from build123d import *

# Parameters (mm, degrees)
F0_R          = 9.525
F1_DEPTH      = 127
F2_R          = 9.525
F3_DEPTH      = 38.1
F3_DEPTH_BACK = 38.1


with BuildPart() as f1:
    # F0 (on Front) → F1 (new body)
    with BuildSketch(Plane.XZ):
        Polygon((-9.525, -23.880164), (-9.525, -36.580164), (9.525, -36.580164), (9.525, -23.880164), (19.05, -23.880164), (19.05, 0), (19.05, 25.4), (0, 25.4), (-19.05, 25.4), (-19.05, 0), (-19.05, -23.880164), align=None)
        Circle(F0_R, mode=Mode.SUBTRACT)
    extrude(amount=F1_DEPTH)

    # F2 (on Right) → F3 (cut, two sides)
    with BuildSketch(Plane.YZ) as f3_sk:
        with Locations((-32.103937, 0)):
            Circle(F2_R)
        with Locations((-95.37492, 0)):
            Circle(F2_R)
    extrude(amount=F3_DEPTH, mode=Mode.SUBTRACT)
    extrude(f3_sk.sketch, amount=-F3_DEPTH_BACK, mode=Mode.SUBTRACT)


solid = f1.part
Verification items for the finished model (mm, model axes). A direction names the side the tool comes from. Give positions to 0.01 mm unless a question says otherwise; leave off trailing zeros. Order: outer loops, then holes, each group sorted by start corner. A loop starts at its lowest first (then second) coordinate and runs counter-clockwise, first axis right, second up. Notation, with made-up numbers: M 44,44 L 66,44 A16 ccw 66,67 Z; hole C -12,-37.5 d4. An arc over 180 degrees is marked long. Answer as a JSON object with one key per item and string values. Group by question number.
1) Cross-section at B-B (y = -18). Enter the section's corners in (x, z) (3 decimals).
2) Access from +Z, -Z, +X, -X, +Y, -Y to the whole of each face (thin tool, end or side, straight path). Record for faces 5 (the face through (-9.525, -63, -30)), 6 (the face through (11.51, -23.02, 2.86)), 7 (the face through (14, -63, -23.88)).
3) Cross-section at A-A (z = 0). Enter the section's corners in (x, y) (3 decimals).
4) Cross-section at C-C (x = 14). Enter the section's corners in (y, z) (3 decimals).
5) Mould release check, pull along X, two halves, no side actions. Record for faces 1 (the face through (-9.516, -63.297, 0.419)), 2 (the face through (-19.05, -63, 1)), 3 (the face through (19.05, -63, 0)), 4 (the face through (0, -63, -36.58)): released by +X, released by -X, zero draft, split by the parting line, or undercut.
6) Cross-section at D-D (x = 6). Enter the section's corners in (y, z) (3 decimals), then the cut area to 3 significant figures.
7) Depth check by flat-ended pin: pin 1 Ø4 at (y, z) = (-71.5, -28) entering from -X (3 decimals); pin 2 Ø5 at (x, y) = (-15, -45.5) entering from -Z; pin 3 Ø14 at (y, z) = (-94.5, -33) entering from +X (3 decimals). Enter the tip coordinate at first touch or a pass-through.
8) Scan lines: line 1 along Y through (x, z) = (-13, 0); line 2 along Z through (x, y) = (0, -83) (3 decimals); line 3 along X through (y, z) = (-45.5, 0) (3 decimals). Record each from-to range of solid material in increasing order. Write a range as [from, to].
Result sheet:
{
 "1": {"outline": "M -19.05,-23.88 L -9.525,-23.88 L -9.525,-36.58 L 9.525,-36.58 L 9.525,-23.88 L 19.05,-23.88 L 19.05,25.4 L -19.05,25.4 Z; hole C 0,0 d19.05"},
 "2": {"face 5": "-Z, -X, +Y, -Y", "face 6": "+X, -X", "face 7": "-Z, +X, +Y, -Y"},
 "3": {"outline": "M -19.05,-127 L -9.525,-127 L -9.525,-104.9 L -19.05,-104.9 Z; M -19.05,-85.85 L -9.525,-85.85 L -9.525,-41.629 L -19.05,-41.629 Z; M -19.05,-22.579 L -9.525,-22.579 L -9.525,0 L -19.05,0 Z; M 9.525,-127 L 19.05,-127 L 19.05,-104.9 L 9.525,-104.9 Z; M 9.525,-85.85 L 19.05,-85.85 L 19.05,-41.629 L 9.525,-41.629 Z; M 9.525,-22.579 L 19.05,-22.579 L 19.05,0 L 9.525,0 Z"},
 "4": {"outline": "M -127,-23.88 L 0,-23.88 L 0,25.4 L -127,25.4 Z; hole C -95.375,0 d19.05; hole C -32.104,0 d19.05"},
 "5": {"face 1": "undercut", "face 2": "released by -X", "face 3": "released by +X", "face 4": "zero draft"},
 "6": {"outline": "M -127,-36.58 L 0,-36.58 L 0,-7.398 L -26.104,-7.398 A9.525 cw -38.104,-7.398 L -89.375,-7.398 A9.525 cw -101.375,-7.398 L -127,-7.398 Z; M -127,7.398 L -101.375,7.398 A9.525 cw -89.375,7.398 L -38.104,7.398 A9.525 cw -26.104,7.398 L 0,7.398 L 0,25.4 L -127,25.4 Z", "area": "5,920 mm2"},
 "7": {"pin 1": "stops at x = -9.525", "pin 2": "stops at z = -23.88", "pin 3": "stops at x = 9.525"},
 "8": {"line 1": "y = [-127, -104.9], [-85.85, -41.63], [-22.58, 0]", "line 2": "z = [-36.58, -9.525], [9.525, 25.4]", "line 3": "x = [-19.05, -9.525], [9.525, 19.05]"}
}
